```python
from build123d import *

# Parameters (mm, degrees)
SKETCH1_W             = 9
SKETCH1_H             = 12
BOSS_EXTRUDE1_DEPTH   = 60
BOSS_EXTRUDE1_2_DEPTH = 60
SKETCH2_W             = 9
SKETCH2_H             = 20
BOSS_EXTRUDE2_DEPTH   = 2
SKETCH3_R             = 1.4
CUT_EXTRUDE1_DEPTH    = 6
FILLET1_R             = 5.5
FILLET2_R             = 5.5
SKETCH4_R             = 1.5
BOSS_EXTRUDE4_DEPTH   = 2
FILLET4_R             = 10


with BuildPart() as part:
    # Sketch1 → Boss-Extrude1 (new body)
    with BuildSketch(Plane(origin=(0, 0, 0), x_dir=(1, 0, 0), z_dir=(0, 1, 0))):
        with Locations((39, 0)):
            Rectangle(SKETCH1_W, SKETCH1_H)
    extrude(amount=BOSS_EXTRUDE1_DEPTH)



with BuildPart() as body_2:
    # Sketch1 → Boss-Extrude1 2 (new body)
    with BuildSketch(Plane(origin=(0, 0, 0), x_dir=(1, 0, 0), z_dir=(0, 1, 0))):
        with Locations((-39, 0)):
            Rectangle(SKETCH1_W, SKETCH1_H)
    extrude(amount=BOSS_EXTRUDE1_2_DEPTH)


with BuildPart() as part_1:
    add(part.part)

    add(body_2.part)  # Boss-Extrude2 merges body 2
    # Sketch2 → Boss-Extrude2 (add)
    with BuildSketch(Plane.XZ):
        with Locations((-39, 0)):
            Rectangle(SKETCH2_W, SKETCH2_H)
        with Locations((39, 0)):
            Rectangle(SKETCH2_W, SKETCH2_H)
    extrude(amount=BOSS_EXTRUDE2_DEPTH)

    # Sketch3 → Cut-Extrude1 (cut)
    with BuildSketch(Plane.XZ.offset(2)):
        with Locations(Location((39, 0, 0), (0, 0, 270))):
            Circle(SKETCH3_R)
        with Locations(Location((-39, 0, 0), (0, 0, 270))):
            Circle(SKETCH3_R)
    extrude(amount=-CUT_EXTRUDE1_DEPTH, mode=Mode.SUBTRACT)

    # Fillet1
    # the kernel refuses this fillet: 5.5 mm, written as the material it adds along each edge
    with BuildSketch(Plane(origin=(-43.5, 0, -6), x_dir=(0, 1, 0), z_dir=(1, 0, 0))) as fillet1_piece_1:
        with BuildLine():
            CenterArc((5.291502622, -5.5), FILLET1_R, 90, 74.173379868)
            Line((0, -4), (-0.105830052, -3.97))
            ThreePointArc((-0.105830052, -3.97), (-0.11, -2), (-0.11, 0))
            Line((-0.11, 0), (0, 0.11))
            Line((0, 0.11), (5.291502622, 0.11))
            Line((5.291502622, 0.11), (5.291502622, 0))
        make_face()
    extrude(amount=9)
    with BuildSketch(Plane(origin=(-34.5, 0, 6), x_dir=(0, 0, 1), z_dir=(-1, 0, 0))) as fillet1_piece_2:
        with BuildLine():
            CenterArc((5.5, 5.291502622), FILLET1_R, 180, 74.173379868)
            Line((0, 5.291502622), (-0.11, 5.291502622))
            Line((-0.11, 5.291502622), (-0.11, 0))
            Line((-0.11, 0), (0, -0.11))
            ThreePointArc((0, -0.11), (2, -0.11), (3.97, -0.105830052))
            Line((3.97, -0.105830052), (4, 0))
        make_face()
    extrude(amount=9)

    # Fillet2
    # the kernel refuses this fillet: 5.5 mm, written as the material it adds along each edge
    with BuildSketch(Plane(origin=(34.5, 0, -6), x_dir=(0, 0, -1), z_dir=(1, 0, 0))) as fillet2_piece_1:
        with BuildLine():
            CenterArc((5.5, 5.291502622), FILLET2_R, 180, 74.173379868)
            Line((0, 5.291502622), (-0.11, 5.291502622))
            Line((-0.11, 5.291502622), (-0.11, 0))
            Line((-0.11, 0), (0, -0.11))
            ThreePointArc((0, -0.11), (2, -0.11), (3.97, -0.105830052))
            Line((3.97, -0.105830052), (4, 0))
        make_face()
    extrude(amount=9)
    with BuildSketch(Plane(origin=(43.5, 0, 6), x_dir=(0, 1, 0), z_dir=(-1, 0, 0))) as fillet2_piece_2:
        with BuildLine():
            CenterArc((5.291502622, -5.5), FILLET2_R, 90, 74.173379868)
            Line((0, -4), (-0.105830052, -3.97))
            ThreePointArc((-0.105830052, -3.97), (-0.11, -2), (-0.11, 0))
            Line((-0.11, 0), (0, 0.11))
            Line((0, 0.11), (5.291502622, 0.11))
            Line((5.291502622, 0.11), (5.291502622, 0))
        make_face()
    extrude(amount=9)

    # Sketch4 → Boss-Extrude4 (add)
    with BuildSketch(Plane(origin=(0, 60, 0), x_dir=(1, 0, 0), z_dir=(0, 1, 0))):
        with BuildLine():
            Line((-55, 30), (55, 30))
            ThreePointArc((55, 30), (58.535533906, 28.535533906), (60, 25))
            Line((60, 25), (60, -25))
            ThreePointArc((60, -25), (58.535533906, -28.535533906), (55, -30))
            Line((55, -30), (-55, -30))
            ThreePointArc((-55, -30), (-58.535533906, -28.535533906), (-60, -25))
            Line((-60, -25), (-60, 25))
            ThreePointArc((-60, 25), (-58.535533906, 28.535533906), (-55, 30))
        make_face()
        with Locations(Location((-57, -2.5, 0), (0, 0, 270))):
            Circle(SKETCH4_R, mode=Mode.SUBTRACT)
        with Locations(Location((-57, -12.5, 0), (0, 0, 270))):
            Circle(SKETCH4_R, mode=Mode.SUBTRACT)
        with Locations(Location((57, -12.5, 0), (0, 0, 270))):
            Circle(SKETCH4_R, mode=Mode.SUBTRACT)
        with Locations(Location((57, -2.5, 0), (0, 0, 270))):
            Circle(SKETCH4_R, mode=Mode.SUBTRACT)
        with Locations(Location((57, 2.5, 0), (0, 0, 270))):
            Circle(SKETCH4_R, mode=Mode.SUBTRACT)
        with Locations(Location((57, 12.5, 0), (0, 0, 270))):
            Circle(SKETCH4_R, mode=Mode.SUBTRACT)
        with Locations(Location((-57, 12.5, 0), (0, 0, 270))):
            Circle(SKETCH4_R, mode=Mode.SUBTRACT)
        with Locations(Location((-57, 2.5, 0), (0, 0, 270))):
            Circle(SKETCH4_R, mode=Mode.SUBTRACT)
        with BuildLine():
            Line((55, 23.5), (10, 23.5))
            ThreePointArc((10, 23.5), (8.5, 25), (10, 26.5))
            Line((10, 26.5), (55, 26.5))
            ThreePointArc((55, 26.5), (56.5, 25), (55, 23.5))
        make_face(mode=Mode.SUBTRACT)
        with BuildLine():
            Line((-55, -23.5), (-10, -23.5))
            ThreePointArc((-10, -23.5), (-8.5, -25), (-10, -26.5))
            Line((-10, -26.5), (-55, -26.5))
            ThreePointArc((-55, -26.5), (-56.5, -25), (-55, -23.5))
        make_face(mode=Mode.SUBTRACT)
        with BuildLine():
            Line((-55, 23.5), (-10, 23.5))
            ThreePointArc((-10, 23.5), (-8.5, 25), (-10, 26.5))
            Line((-10, 26.5), (-55, 26.5))
            ThreePointArc((-55, 26.5), (-56.5, 25), (-55, 23.5))
        make_face(mode=Mode.SUBTRACT)
        with BuildLine():
            Line((55, -23.5), (10, -23.5))
            ThreePointArc((10, -23.5), (8.5, -25), (10, -26.5))
            Line((10, -26.5), (55, -26.5))
            ThreePointArc((55, -26.5), (56.5, -25), (55, -23.5))
        make_face(mode=Mode.SUBTRACT)
    extrude(amount=BOSS_EXTRUDE4_DEPTH)

    # Fillet4
    fillet4_edges = [part_1.edges().sort_by_distance(p)[0] for p in [
        (39, 60, 6),
        (39, 60, -6),
        (-39, 60, -6),
        (-39, 60, 6),
    ]]
    fillet(fillet4_edges, radius=FILLET4_R)


solid = part_1.part
```
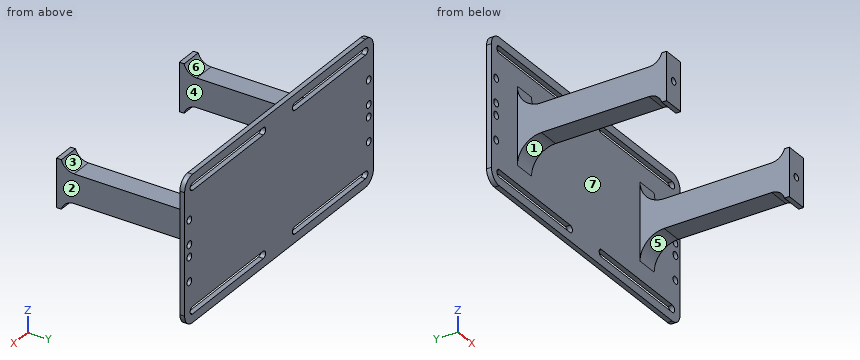
Verification items for the finished model (mm, model axes). Face numbers are marked on the shaded views. A direction names the side the tool comes from. Coordinates: 2 decimals unless noted, no trailing zeros. Write each loop counter-clockwise with the first axis right and the second up, starting at its lowest first coordinate (ties: lowest second). Pieces come first, ordered by that corner, then holes. Notation, with made-up numbers: (29, 71) - (59, 71) arc R27 cw to (59, 91) - close; hole circle Ø10 at (-33, -23). An arc over 180 degrees is marked (long way). Write item = value, one per line.
Q1. Material ranges on L1, parallel to X at y = 60.55, z = 2.5; L2, parallel to X at y = -0.15, z = 0; L3, parallel to Y at x = -47.5, z = -12.5, recorded low to high. Write a range as from..to.
Answer:
L1 = -60..-58.5, -55.5..55.5, 58.5..60
L2 = -43.5..-40.4, -37.6..-34.5, 34.5..37.6, 40.4..43.5
L3 = 60..62
Q2. Cross-section at C-C (z = -12.5). Enter the section's corners in (x, y).
Answer:
outline = (-60, 60) - (-58.5, 60) - (-58.5, 62) - (-60, 62) - close; (-55.5, 60) - (-43.5, 60) - (-43.5, 59.37) - (-34.5, 59.37) - (-34.5, 60) - (34.5, 60) - (34.5, 59.37) - (43.5, 59.37) - (43.5, 60) - (55.5, 60) - (55.5, 62) - (-55.5, 62) - close; (58.5, 60) - (60, 60) - (60, 62) - (58.5, 62) - close
Q3. Mould release check, pull along Y, two halves, no side actions. Record for the marked faces 4, 5, 6 and 7: released by +Y, released by -Y, zero draft, split by the parting line, or undercut.
Answer:
face_4 = zero draft
face_5 = undercut
face_6 = undercut
face_7 = released by -Y
Q4. Cross-section at D-D (x = 24.5). Enter the section's corners in (y, z).
Answer:
outline = (60, -30) - (62, -30) - (62, -26.5) - (60, -26.5) - close; (60, -23.5) - (62, -23.5) - (62, 23.5) - (60, 23.5) - close; (60, 26.5) - (62, 26.5) - (62, 30) - (60, 30) - close
Q5. Go/stop test with flat-tipped pins: pin 1 Ø8 at (y, z) = (42, -5) entering from +X; pin 2 Ø5 at (x, z) = (-57, -2.5) entering from +Y; pin 3 Ø9.5 at (y, z) = (40.5, -5) entering from -X; pin 4 Ø1 at (x, z) = (-16, -14) entering from -Y. Record where each tip stops, or that it passes through.
Answer:
pin_1 = 43.5
pin_2 = 62
pin_3 = -43.5
pin_4 = 60
Q6. Cross-section at B-B (y = 40.5). Enter the section's corners in (x, z), plus the area to 3 significant figures.
Answer:
outline = (-43.5, -6) - (-34.5, -6) - (-34.5, 6) - (-43.5, 6) - close; (34.5, -6) - (43.5, -6) - (43.5, 6) - (34.5, 6) - close
area = 216 mm²
Q7. Cross-section at A-A (x = 39). Enter the section's corners in (y, z).
Answer:
outline = (-2, -10) - (0, -10) arc R5.5 cw to (5.29, -6) - (50, -6) arc R10 cw to (60, -16) - (60, -23.5) - (62, -23.5) - (62, 23.5) - (60, 23.5) - (60, 16) arc R10 cw to (50, 6) - (5.29, 6) arc R5.5 cw to (0, 10) - (-2, 10) - (-2, 1.4) - (4, 1.4) - (4, -1.4) - (-2, -1.4) - close; (60, -30) - (62, -30) - (62, -26.5) - (60, -26.5) - close; (60, 26.5) - (62, 26.5) - (62, 30) - (60, 30) - close
Q8. Access from +Z, -Z, +X, -X, +Y, -Y to the whole of each face (thin tool, end or side, straight path). Record for the marked faces 1, 2 and 3.
Answer:
face_1 = -Z, +X, -X
face_2 = +Z, -Z, +X, -Y
face_3 = +Z, +X, -X
